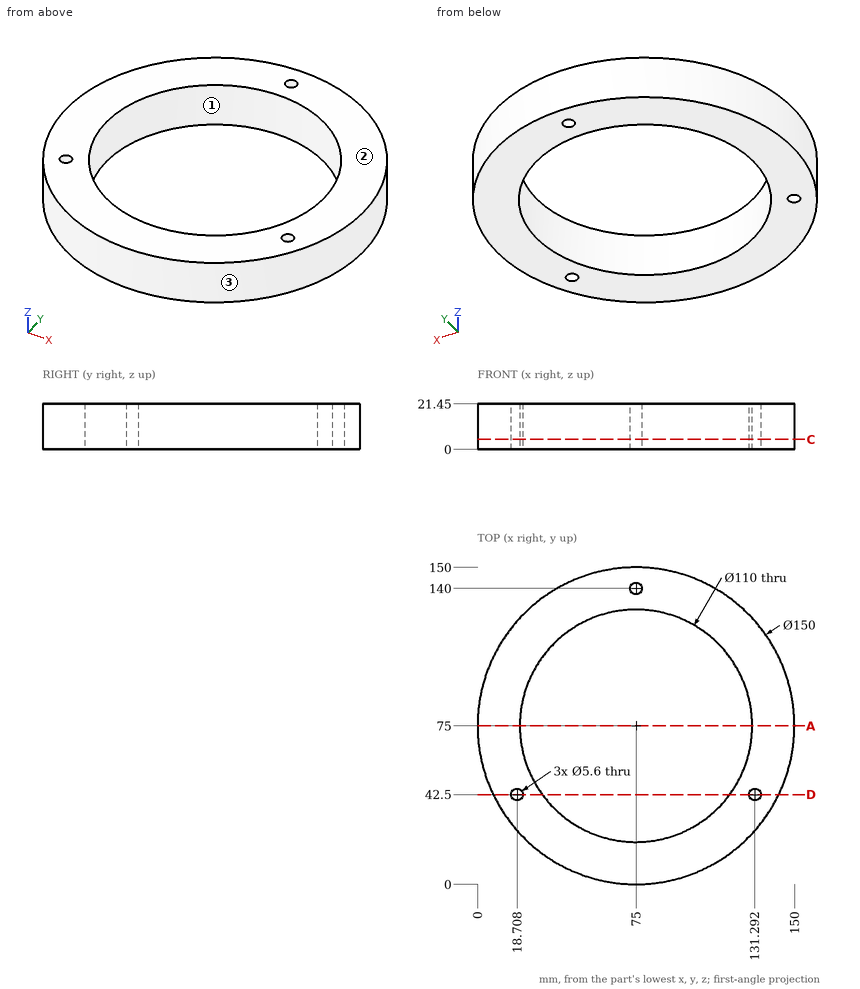
Can you work these out from the drawing? Everything is in mm from the part's minimum corner. Coordinates: 2 decimals unless noted, no trailing zeros. Loops run counter-clockwise (first coordinate to the right, second up) from the corner with the lowest first, then second, coordinate; pieces in that order, holes last. Notation, with made-up numbers: M -18,10 L 41,10 A25 ccw 41,39 Z; hole C -33,39 d4. An arc over 180 degrees is marked long. Put each result on its own line as item: value. Start each with the question number.
(1) Thinking about a two-plate mould opening in X: for the marked faces 1, 2 and 3, which applies, pulls with the +X half, pulls with the -X half, needs draft (parallel to the pull), parting line crosses it, or undercut?
(2) Suppose I cut it at D-D on y = 42.5. Please give me the cut outline in (x, z), then the cut area to 3 significant figures.
(3) I need wall thicknesses on line 1 (Y direction, x = 75, z = 10.75); line 2 (X direction, y = 24, z = 10) (1 decimal); line 3 (Y direction, x = 67, z = 7.25) (1 decimal). Which ranges of each line are inside material? Lowest first, please. Write a range as from..to.
(4) Suppose I cut it at A-A on y = 75. Please give me the cut outline in (x, z).
(5) Will these pins go through, and if not, where does the flat tip stop? P1, Ø1.5, axis at x = 33, z = 15.5, coming from the -Y side; P2, Ø7.5, axis at x = 18.71, y = 42.5, coming from the -Z side; P3, Ø6, axis at y = 85, z = 11, coming from the +X side; P4, Ø5, axis at x = 75, y = 140, coming from the -Z side.
(6) Suppose I cut it at C-C on z = 4.75. Please give me the cut outline in (x, y).
Solutions:
1. face 1: undercut
1. face 2: needs draft
1. face 3: parting line crosses it
2. outline: M 7.41,0 L 15.91,0 L 15.91,21.45 L 7.41,21.45 Z; M 21.51,0 L 30.63,0 L 30.63,21.45 L 21.51,21.45 Z; M 119.37,0 L 128.49,0 L 128.49,21.45 L 119.37,21.45 Z; M 134.09,0 L 142.59,0 L 142.59,21.45 L 134.09,21.45 Z
2. area: 756 mm2
3. line 1: y = 0..20, 130..137.2, 142.8..150
3. line 2: x = 20..54.4, 95.6..130
3. line 3: y = 0.4..20.6, 129.4..149.6
4. outline: M 0,0 L 20,0 L 20,21.45 L 0,21.45 Z; M 130,0 L 150,0 L 150,21.45 L 130,21.45 Z
5. P1: stops at y = 12.36
5. P2: stops at z = 0
5. P3: stops at x = 149.67
5. P4: passes through
6. outline: C 75,75 d150; hole C 18.71,42.5 d5.6; hole C 75,75 d110; hole C 75,140 d5.6; hole C 131.29,42.5 d5.6
